from build123d import *

# Parameters (mm, degrees)
SKETCH1_R           = 2.65
SKETCH1_W           = 40
SKETCH1_H           = 15
BOSS_EXTRUDE1_DEPTH = 10
CUT_EXTRUDE2_DEPTH  = 10
BOSS_EXTRUDE3_DEPTH = 43
CUT_EXTRUDE3_REACH  = 143.262
SKETCH13_R          = 11
SKETCH13_R_2        = 1.65
SKETCH15_W          = 3.5
SKETCH15_H          = 23.85
BOSS_EXTRUDE4_DEPTH = 43
SKETCH16_W          = 42.5
SKETCH16_H          = 3.5
BOSS_EXTRUDE5_DEPTH = 10


with BuildPart() as part:
    # Sketch1 → Boss-Extrude1 (new body)
    with BuildSketch(Plane(origin=(0, 0, 0), x_dir=(1, 0, 0), z_dir=(0, 1, 0))):
        Polygon((51, 85.65), (48, 85.65), (48, 62.5), (26, 62.5), (26, 0), (125, 0), (125, 62.5), (103, 62.5), (103, 85.65), (100, 85.65), align=None)
        with Locations(Location((108.05464, 46.5, 0), (0, 0, 270))):
            Circle(SKETCH1_R, mode=Mode.SUBTRACT)
        with Locations(Location((41.87366, 46.5, 0), (0, 0, 270))):
            Circle(SKETCH1_R, mode=Mode.SUBTRACT)
        with Locations(Location((41.87366, 16, 0), (0, 0, 270))):
            Circle(SKETCH1_R, mode=Mode.SUBTRACT)
        with Locations(Location((108.05464, 16, 0), (0, 0, 270))):
            Circle(SKETCH1_R, mode=Mode.SUBTRACT)
        with Locations((75.5, 31.15)):
            Rectangle(SKETCH1_W, SKETCH1_H, mode=Mode.SUBTRACT)
    extrude(amount=BOSS_EXTRUDE1_DEPTH)

    # Sketch8 → Cut-Extrude2 (cut)
    with BuildSketch(Plane(origin=(0, 10, 0), x_dir=(1, 0, 0), z_dir=(0, 1, 0))):
        Polygon((96.75, 70.488685564), (96.75, 62.5), (103, 62.5), (103, 85.65), (48, 85.65), (48, 62.5), (54.25, 62.5), (54.25, 70.488685564), (54.25, 77.65), (76, 77.65), (96.75, 77.65), align=None)
    extrude(amount=-CUT_EXTRUDE2_DEPTH, mode=Mode.SUBTRACT)

    # Sketch12 → Boss-Extrude3 (add)
    with BuildSketch(Plane(origin=(0, 10, 0), x_dir=(1, 0, 0), z_dir=(0, 1, 0))):
        Polygon((96.75, 42.15), (54.25, 42.15), (54.25, 38.65), (55.5, 38.65), (95.5, 38.65), (96.75, 38.65), align=None)
    extrude(amount=BOSS_EXTRUDE3_DEPTH)

    # Sketch13 → Cut-Extrude3 (cut, up to next)
    with BuildSketch(Plane.XY.offset(-38.65), mode=Mode.PRIVATE) as cut_extrude3_sk1:
        with Locations((75.5, 31)):
            Circle(SKETCH13_R)
    cut_extrude3_tool1 = extrude(cut_extrude3_sk1.sketch, amount=-CUT_EXTRUDE3_REACH, mode=Mode.PRIVATE) & part.part
    # Sketch13 → Cut-Extrude3 (cut, up to next)
    with BuildSketch(Plane.XY.offset(-38.65), mode=Mode.PRIVATE) as cut_extrude3_sk2:
        with Locations((60, 46.5)):
            Circle(SKETCH13_R_2)
    cut_extrude3_tool2 = extrude(cut_extrude3_sk2.sketch, amount=-CUT_EXTRUDE3_REACH, mode=Mode.PRIVATE) & part.part
    # Sketch13 → Cut-Extrude3 (cut, up to next)
    with BuildSketch(Plane.XY.offset(-38.65), mode=Mode.PRIVATE) as cut_extrude3_sk3:
        with Locations((91, 46.5)):
            Circle(SKETCH13_R_2)
    cut_extrude3_tool3 = extrude(cut_extrude3_sk3.sketch, amount=-CUT_EXTRUDE3_REACH, mode=Mode.PRIVATE) & part.part
    # Sketch13 → Cut-Extrude3 (cut, up to next)
    with BuildSketch(Plane.XY.offset(-38.65), mode=Mode.PRIVATE) as cut_extrude3_sk4:
        with Locations((91, 15.5)):
            Circle(SKETCH13_R_2)
    cut_extrude3_tool4 = extrude(cut_extrude3_sk4.sketch, amount=-CUT_EXTRUDE3_REACH, mode=Mode.PRIVATE) & part.part
    # Sketch13 → Cut-Extrude3 (cut, up to next)
    with BuildSketch(Plane.XY.offset(-38.65), mode=Mode.PRIVATE) as cut_extrude3_sk5:
        with Locations((60, 15.5)):
            Circle(SKETCH13_R_2)
    cut_extrude3_tool5 = extrude(cut_extrude3_sk5.sketch, amount=-CUT_EXTRUDE3_REACH, mode=Mode.PRIVATE) & part.part
    add(cut_extrude3_tool1.solids().sort_by_distance((75.5, 31, -38.65))[0], mode=Mode.SUBTRACT)
    add(cut_extrude3_tool2.solids().sort_by_distance((60, 46.5, -38.65))[0], mode=Mode.SUBTRACT)
    add(cut_extrude3_tool3.solids().sort_by_distance((91, 46.5, -38.65))[0], mode=Mode.SUBTRACT)
    add(cut_extrude3_tool4.solids().sort_by_distance((91, 15.5, -38.65))[0], mode=Mode.SUBTRACT)
    add(cut_extrude3_tool5.solids().sort_by_distance((60, 15.5, -38.65))[0], mode=Mode.SUBTRACT)

    # Sketch15 → Boss-Extrude4 (add)
    with BuildSketch(Plane(origin=(0, 10, 0), x_dir=(1, 0, 0), z_dir=(0, 1, 0))):
        with Locations((98.5, 50.575)):
            Rectangle(SKETCH15_W, SKETCH15_H)
        with Locations((52.5, 50.575)):
            Rectangle(SKETCH15_W, SKETCH15_H)
    extrude(amount=BOSS_EXTRUDE4_DEPTH)

    # Sketch16 → Boss-Extrude5 (add)
    with BuildSketch(Plane(origin=(0, 10, 0), x_dir=(1, 0, 0), z_dir=(0, 1, 0))):
        with Locations((75.5, 79.4)):
            Rectangle(SKETCH16_W, SKETCH16_H)
    extrude(amount=-BOSS_EXTRUDE5_DEPTH)


solid = part.part
Can you work these out from the model? Positions are in its coordinate system, mm. A direction names the side the tool comes from. Coordinates: 2 decimals unless noted, no trailing zeros. Loops run counter-clockwise (first coordinate to the right, second up) from the corner with the lowest first, then second, coordinate; pieces in that order, holes last. Notation, with made-up numbers: (37.25, 76) - (42.25, 76) arc R29 cw to (42.25, 114) - close; hole circle Ø7 at (22.25, -39). An arc over 180 degrees is marked (long way). Answer as a JSON object with one key per item and string values. Group by question number.
Item 1: For pin 1 (7 mm diameter, centred on x = 108.05, z = -46.5, fed in from +Y); pin 2 (8 mm diameter, centred on x = 87.5, y = 16, fed in from +Z); pin 3 (22.5 mm diameter, centred on x = 44, y = 35, fed in from -Z), each with a flat end and sliding along its axis, tell me the tip position at first contact or that it passes through.
Item 2: If we mould it in two halves opening along Y, with no side actions, what happens to faces 6 (the face through (40.26, 4.93, -48.6)), 7 (the face through (75, 0, -41)), 8 (the face through (89.784, 47.615, -40.375))? For each: released by +Y, released by -Y, zero draft, split by the parting line, or undercut.
Item 3: If we section it at C-C (x = 60): List the corners of the cut face in (y, z) for me, plus the area to 3 significant figures.
Item 4: If we section it at A-A (z = -16): List the corners of the cut face in (x, y) for me.
Item 5: If we section it at B-B (y = 31): List the corners of the cut face in (x, z) for me, plus the area to 3 significant figures.
Item 6: If I drill on L1, parallel to Y at x = 91, z = -41; L2, parallel to X at y = 19, z = -61.5; L3, parallel to Z at x = 73, y = 48, over which ranges is the centre line in solid material (lowest first)? Write a range as from..to.
Item 7: If we section it at D-D (y = 46.5): List the corners of the cut face in (x, z) for me, plus the area to 3 significant figures.
Item 8: On a 3-axis mill with a long thin cutter (end or side, diameter ignored), from which of +Z, -Z, +X, -X, +Y, -Y can I reach the whole of each face in a straight line? I mean faces 1 (the face through (108, 9, -62.5)), 2 (the face through (55.5, 5, -31)), 3 (the face through (50.75, 31, -50)), 4 (the face through (54.25, 5, -72)), 5 (the face through (66, 22, -42.15)). Say none if no direction works.
Returned:
{
 "1": {"pin 1": "stops at y = 10", "pin 2": "stops at z = -38.65", "pin 3": "stops at z = -62.5"},
 "2": {"face 6": "zero draft", "face 7": "released by -Y", "face 8": "undercut"},
 "3": {"outline": "(0, -81.15) - (10, -81.15) - (10, -42.15) - (13.85, -42.15) - (13.85, -38.65) - (0, -38.65) - close; (0, -23.65) - (10, -23.65) - (10, 0) - (0, 0) - close; (17.15, -42.15) - (44.85, -42.15) - (44.85, -38.65) - (17.15, -38.65) - close; (48.15, -42.15) - (53, -42.15) - (53, -38.65) - (48.15, -38.65) - close", "area": "789 mm²"},
 "4": {"outline": "(26, 0) - (39.22, 0) - (39.22, 10) - (26, 10) - close; (44.52, 0) - (105.4, 0) - (105.4, 10) - (44.52, 10) - close; (110.7, 0) - (125, 0) - (125, 10) - (110.7, 10) - close"},
 "5": {"outline": "(50.75, -62.5) - (54.25, -62.5) - (54.25, -42.15) - (64.5, -42.15) - (64.5, -38.65) - (50.75, -38.65) - close; (86.5, -42.15) - (96.75, -42.15) - (96.75, -62.5) - (100.25, -62.5) - (100.25, -38.65) - (86.5, -38.65) - close", "area": "239 mm²"},
 "6": {"L1": "y = 0..13.85, 17.15..44.85, 48.15..53", "L2": "x = 50.75..54.25, 96.75..100.25", "L3": "z = -42.15..-38.65"},
 "7": {"outline": "(50.75, -62.5) - (54.25, -62.5) - (54.25, -42.15) - (58.35, -42.15) - (58.35, -38.65) - (50.75, -38.65) - close; (61.65, -42.15) - (89.35, -42.15) - (89.35, -38.65) - (61.65, -38.65) - close; (92.65, -42.15) - (96.75, -42.15) - (96.75, -62.5) - (100.25, -62.5) - (100.25, -38.65) - (92.65, -38.65) - close", "area": "293 mm²"},
 "8": {"face 1": "-Z, +X, +Y, -Y", "face 2": "+Y, -Y", "face 3": "+Z, -Z, -X, +Y", "face 4": "-Z, -X, +Y, -Y", "face 5": "-Z, +Y"}
}
